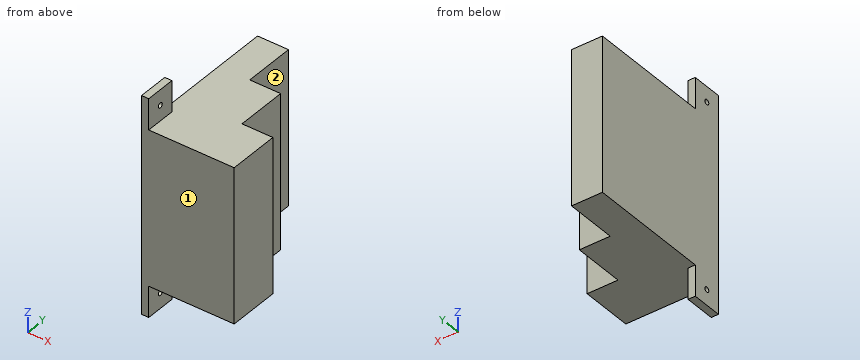
```python
from build123d import *

# Parameters (mm, degrees)
BOSS_EXTRUDE1_DEPTH = 190.5
SKETCH2_W           = 76.2
SKETCH2_H           = 76.2
SKETCH2_R           = 6.35
BOSS_EXTRUDE2_DEPTH = 17.78


with BuildPart() as part:
    # Sketch1 → Boss-Extrude1 (new, symmetric)
    with BuildSketch(Plane.XY):
        Polygon((0, 0), (0, 381), (76.2, 381), (76.2, 254), (152.4, 254), (152.4, 127), (228.6, 127), (228.6, 0), align=None)
    extrude(amount=BOSS_EXTRUDE1_DEPTH, both=True)

    # Sketch2 → Boss-Extrude2 (add)
    # profile 1 of 2: a face of its own
    with BuildSketch(Plane.ZY):
        with Locations((228.6, 38.1)):
            Rectangle(SKETCH2_W, SKETCH2_H)
        with Locations((228.6, 38.1)):
            Circle(SKETCH2_R, mode=Mode.SUBTRACT)
    # profile 2 of 2: a face of its own
    with BuildSketch(Plane.ZY):
        with Locations((-228.6, 38.1)):
            Rectangle(SKETCH2_W, SKETCH2_H)
        with Locations((-228.6, 38.1)):
            Circle(SKETCH2_R, mode=Mode.SUBTRACT)
    extrude(amount=-BOSS_EXTRUDE2_DEPTH)


solid = part.part
```
CAD build for the part. Positions are in the model's coordinates, mm. Face numbers are marked on the shaded views. A direction names the side the tool comes from. Coordinates: 2 decimals unless noted, no trailing zeros. Loops run counter-clockwise (first coordinate to the right, second up) from the corner with the lowest first, then second, coordinate; pieces in that order, holes last. Notation, with made-up numbers: (29, 58) - (47, 58) arc R23 cw to (47, 93) - close; hole circle Ø9 at (-31.75, 28). An arc over 180 degrees is marked (long way). Return JSON: item names as keys, results as strings.
1. 3-axis set-ups, long thin cutter, end or side, ignore diameter. For the marked faces 1 and 2: which of +Z, -Z, +X, -X, +Y, -Y reach the whole face in a straight line?
Result:
{"face 1": "+Z, -Z, +X, -X, -Y", "face 2": "+Z, -Z, +X, +Y"}
2. Band-saw the part on C-C (z = -91). Give the cut face in (x, y), and give its area (3 significant figures).
Result:
{"outline": "(0, 0) - (228.6, 0) - (228.6, 127) - (152.4, 127) - (152.4, 254) - (76.2, 254) - (76.2, 381) - (0, 381) - close", "area": "58,100 mm2"}
3. Band-saw the part on D-D (x = 213). Give the cut face in (y, z).
Result:
{"outline": "(0, -190.5) - (127, -190.5) - (127, 190.5) - (0, 190.5) - close"}
4. Band-saw the part on B-B (y = 38.1). Give the cut face in (x, z).
Result:
{"outline": "(0, -266.7) - (17.78, -266.7) - (17.78, -234.95) - (0, -234.95) - close; (0, -222.25) - (17.78, -222.25) - (17.78, -190.5) - (228.6, -190.5) - (228.6, 190.5) - (17.78, 190.5) - (17.78, 222.25) - (0, 222.25) - close; (0, 234.95) - (17.78, 234.95) - (17.78, 266.7) - (0, 266.7) - close"}
5. Band-saw the part on A-A (z = 228.6). Give the cut face in (x, y).
Result:
{"outline": "(0, 0) - (17.78, 0) - (17.78, 31.75) - (0, 31.75) - close; (0, 44.45) - (17.78, 44.45) - (17.78, 76.2) - (0, 76.2) - close"}
6. Probe L1, parallel to Z at x = 11, y = 38; L2, parallel to Y at x = 8.25, z = 228.6; L3, parallel to X at y = 221.5, z = -126.5. List the from-to ranges inside material, lowest first. Write a range as from..to.
Result:
{"L1": "z = -266.7..-234.95, -222.25..222.25, 234.95..266.7", "L2": "y = 0..31.75, 44.45..76.2", "L3": "x = 0..152.4"}
7. Drop flat-ended pins along their axis: pin 1 (5 mm diameter, centred on x = 153.5, z = 167, fed in from -Y); pin 2 (14 mm diameter, centred on x = 4.5, z = -243, fed in from +Y); pin 3 (2 mm diameter, centred on x = 105, z = 127.5, fed in from +Y); pin 4 (23 mm diameter, centred on y = 46.5, z = -209.5, fed in from +X). Give the stop position or say it passes through.
Result:
{"pin 1": "stops at y = 0", "pin 2": "stops at y = 76.2", "pin 3": "stops at y = 254", "pin 4": "stops at x = 17.78"}
